```python
from build123d import *

# Parameters (mm, degrees)
SKETCH1_W                      = 73
SKETCH1_H                      = 93
BOSS_EXTRUDE1_DEPTH            = 47
SKETCH2_R                      = 17
BOSS_EXTRUDE2_DEPTH            = 3.4
SKETCH3_R                      = 9
BOSS_EXTRUDE3_DEPTH            = 33.6
SKETCH4_R                      = 3
CUT_EXTRUDE1_DEPTH             = 3
M8X1_0_TAPPED_HOLE1_AT_2_COUNT = 2
M8X1_0_TAPPED_HOLE1_AT_2_PITCH = 50
M8X1_0_TAPPED_HOLE2_D          = 7
M8X1_0_TAPPED_HOLE2_DEPTH      = 19
M8X1_0_TAPPED_HOLE2_TIP        = 2.103012167


with BuildPart() as part:
    # Sketch1 → Boss-Extrude1 (new, symmetric)
    with BuildSketch(Plane.XY):
        with Locations((0, 11)):
            Rectangle(SKETCH1_W, SKETCH1_H)
    extrude(amount=BOSS_EXTRUDE1_DEPTH, both=True)

    # Sketch2 → Boss-Extrude2 (add)
    with BuildSketch(Plane.XY.offset(47)):
        Circle(SKETCH2_R)
    boss_extrude2 = extrude(amount=BOSS_EXTRUDE2_DEPTH)

    # Sketch3 → Boss-Extrude3 (add)
    with BuildSketch(Plane.XY.offset(50.4)):
        Circle(SKETCH3_R)
    boss_extrude3 = extrude(amount=BOSS_EXTRUDE3_DEPTH)

    # Sketch4 → Cut-Extrude1 (cut)
    with BuildSketch(Plane(origin=(0, 9, 0), x_dir=(1, 0, 0), z_dir=(0, 1, 0))):
        with BuildLine():
            ThreePointArc((3, -65), (0, -68), (-3, -65))
            Line((-3, -65), (-3, -84))
            Line((-3, -84), (3, -84))
            Line((3, -84), (3, -65))
        make_face()
        with Locations((0, -65)):
            Circle(SKETCH4_R)
    cut_extrude1 = extrude(amount=-CUT_EXTRUDE1_DEPTH, mode=Mode.SUBTRACT)

    # Sketch6 → M8x1.0 Tapped Hole1 (revolve, cut)
    with BuildSketch(Plane(origin=(-25, 41.5, 47), x_dir=(0, -1, 0), z_dir=(1, 0, 0))):
        Polygon((0, 0), (0, 10.103012167), (3.5, 8), (3.5, 0), align=None)
    m8x1_0_tapped_hole1 = revolve(axis=Axis((-25, 41.5, 53.35), (0, 0, -1)), mode=Mode.SUBTRACT)

    # M8x1.0 Tapped Hole1 at 2: M8x1.0 Tapped Hole1 ×2
    with Locations(*[(i * M8X1_0_TAPPED_HOLE1_AT_2_PITCH, 0, 0) for i in range(1, M8X1_0_TAPPED_HOLE1_AT_2_COUNT)]):
        add(m8x1_0_tapped_hole1, mode=Mode.SUBTRACT)

    # Mirror1: Boss-Extrude2, Boss-Extrude3, Cut-Extrude1, M8x1.0 Tapped Hole1 across plane
    add(boss_extrude2.mirror(Plane.XY))
    add(boss_extrude3.mirror(Plane.XY))
    add(cut_extrude1.mirror(Plane.XY), mode=Mode.SUBTRACT)
    add(m8x1_0_tapped_hole1.mirror(Plane.XY), mode=Mode.SUBTRACT)

    # Mirror1 copy 1 sketch → Mirror1 copy 1 (revolve, cut)
    with BuildSketch(Plane(origin=(25, 41.5, -47), x_dir=(0, -1, 0), z_dir=(1, 0, 0))):
        Polygon((0, 0), (0, -10.103012167), (3.5, -8), (3.5, 0), align=None)
    revolve(axis=Axis((25, 41.5, -53.35), (0, 0, -1)), mode=Mode.SUBTRACT)

    # M8x1.0 Tapped Hole2
    with Locations(Plane(origin=(26.5, -35.5, 26.5), x_dir=(0, 0, -1), z_dir=(0, -1, 0))):
        with Locations((0, 0), (53, 0), (53, -53), (0, -53)):
            Hole(M8X1_0_TAPPED_HOLE2_D / 2, depth=M8X1_0_TAPPED_HOLE2_DEPTH)
            with Locations((0, 0, -(M8X1_0_TAPPED_HOLE2_DEPTH + M8X1_0_TAPPED_HOLE2_TIP / 2))):  # 118° drill point
                Cone(0, M8X1_0_TAPPED_HOLE2_D / 2, M8X1_0_TAPPED_HOLE2_TIP, mode=Mode.SUBTRACT)


solid = part.part
```
Input: part model. Units: mm. Frame: model coordinates. A direction names the side the tool comes from. Round coordinates to 2 decimals unless told otherwise and drop trailing zeros. Loops run counter-clockwise (first coordinate to the right, second up) from the corner with the lowest first, then second, coordinate; pieces in that order, holes last. Notation, with made-up numbers: M 87.25,46 L 123.25,46 A7 ccw 123.25,52 Z; hole C 44,77.25 d10. An arc over 180 degrees is marked long. Answer in a Markdown table with one row per item. Add a question column.
1. Contact query for flat-ended pins moving along their axis: pin 1 (10 mm diameter, centred on y = -9, z = 58, fed in from +X); pin 2 (2 mm diameter, centred on x = 3, z = -61.5, fed in from -Y); pin 3 (5 mm diameter, centred on x = -26, y = -16, fed in from +Z); pin 4 (4 mm diameter, centred on x = 2.5, y = 9.5, fed in from -Z). Output: stop coordinate, or through.
2. Mould query, pull axis X, two halves, no side actions, for faces 4 (the face through (7, -7, -50.4)), 5 (the face through (-36.5, 10, 1)), 6 (the face through (-25, 45, 43)). Classes: released by +X, released by -X, zero draft, split by the parting line, or undercut.
3. Section A-A (x = 0). Output: boundary loops of the cut face in (y, z).
4. Set-up query: faces 1 (the face through (7, -7, 50.4)), 2 (the face through (-1.951, -8.786, -66.965)), 3 (the face through (-23.03, -25.87, 26.04)). Return all of +Z, -Z, +X, -X, +Y, -Y with unobstructed straight access to the full face (end or side cutting, diameter ignored); none if empty.
5. Section C-C (x = -15). Output: boundary loops of the cut face in (y, z).
6. Ray query, probe 1 along X at (y, z) = (-25.5, 26.5); probe 2 along X at (y, z) = (41, -41); probe 3 along Z at (x, y) = (26, -26). Return the intervals inside material, ascending.
7. Section B-B (y = -5). Output: boundary loops of the cut face in (x, z), and give its area (3 significant figures).
8. Section D-D (y = 11). Output: boundary loops of the cut face in (x, z), and give its area (3 significant figures).
Values follow:
| question | item | result |
|---|---|---|
| 1 | pin 1 | x = 8.06 |
| 1 | pin 2 | y = -8.77 |
| 1 | pin 3 | z = 47 |
| 1 | pin 4 | z = -84 |
| 2 | face 4 | zero draft |
| 2 | face 5 | released by -X |
| 2 | face 6 | undercut |
| 3 | outline | M -35.5,-47 L -17,-47 L -17,-50.4 L -9,-50.4 L -9,-84 L 6,-84 L 6,-62 L 9,-62 L 9,-50.4 L 17,-50.4 L 17,-47 L 57.5,-47 L 57.5,47 L 17,47 L 17,50.4 L 9,50.4 L 9,62 L 6,62 L 6,84 L -9,84 L -9,50.4 L -17,50.4 L -17,47 L -35.5,47 Z |
| 4 | face 1 | +Z |
| 4 | face 2 | -Z |
| 4 | face 3 | -Y |
| 5 | outline | M -35.5,-47 L -8,-47 L -8,-50.4 L 8,-50.4 L 8,-47 L 57.5,-47 L 57.5,47 L 8,47 L 8,50.4 L -8,50.4 L -8,47 L -35.5,47 Z |
| 6 | probe 1 | -36.5 to -30, -23 to 23, 30 to 36.5 |
| 6 | probe 2 | -36.5 to -28.46, -21.54 to 21.54, 28.46 to 36.5 |
| 6 | probe 3 | -47 to -29.96, -23.04 to 23.04, 29.96 to 47 |
| 7 | outline | M -36.5,-47 L -16.25,-47 L -16.25,-50.4 L -7.48,-50.4 L -7.48,-84 L 7.48,-84 L 7.48,-50.4 L 16.25,-50.4 L 16.25,-47 L 36.5,-47 L 36.5,47 L 16.25,47 L 16.25,50.4 L 7.48,50.4 L 7.48,84 L -7.48,84 L -7.48,50.4 L -16.25,50.4 L -16.25,47 L -36.5,47 Z |
| 7 | area | 8,090 mm^2 |
| 8 | outline | M -36.5,-47 L -12.96,-47 L -12.96,-50.4 L 12.96,-50.4 L 12.96,-47 L 36.5,-47 L 36.5,47 L 12.96,47 L 12.96,50.4 L -12.96,50.4 L -12.96,47 L -36.5,47 Z |
| 8 | area | 7,040 mm^2 |
